Read the model definition and answer for the solid it produces. Units are mm, in the model's axes. Coordinates: 2 decimals unless noted, no trailing zeros. Loops run counter-clockwise (first coordinate to the right, second up) from the corner with the lowest first, then second, coordinate; pieces in that order, holes last. Notation, with made-up numbers: (-24.5, 24.5) -> (-17.5, 24.5) arc R37 cw to (-17.5, 61.5) -> close; hole circle Ø3 at (24, -11.75). An arc over 180 degrees is marked (long way). Answer as a JSON object with one key per item and string values. Group by question number.
1) Section D-D, the plane x = 25 is taken. Give the vertices of the cut face in (y, z).
2) Consider probe 1 along Y at (x, z) = (0, 5.75); probe 2 along Y at (x, z) = (25, 4); probe 3 along X at (y, z) = (5, 4). Determine where each line is inside the solid, lowest interval first. Write a range as [from, to].
3) Section C-C, the plane y = 2 is taken. Give the vertices of the cut face in (x, z), plus the area to 3 significant figures.
4) Section A-A, the plane z = 4.25 is taken. Give the vertices of the cut face in (x, y).
5) Flat-ended cylindrical pins translate along their axes: P1, Ø8, axis at x = 25, y = 0, coming from the -Z side; P2, Ø5.5, axis at x = -25, y = 0, coming from the +Z side. Find the tip coordinate at first contact, or state that the pin passes through.
6) Section B-B, the plane x = 0 is taken. Give the vertices of the cut face in (y, z).
7) Determine the mould class of faces 1 (the face through (22, 0, 6)), 2 (the face through (-35, 0, 6)), 3 (the face through (0, -19, 6)), 4 (the face through (0, 19, 6)) for opening direction Y: released by +Y, released by -Y, zero draft, split by the parting line, or undercut.
from build123d import *

# Parameters (mm, degrees)
CYLINDER004_R     = 7.5
CYLINDER004_DEPTH = 10
CYLINDER003_R     = 3
CYLINDER003_DEPTH = 10
ARRAY001_X_COUNT  = 2
ARRAY001_X_PITCH  = 50
RECTANGLE001_W    = 70
RECTANGLE001_H    = 38
EXTRUDE001_DEPTH  = 10


with BuildPart() as cilindro004:
    # Cylinder004 → Cylinder004 (new body)
    with BuildSketch(Plane(origin=(0, -5, 0), x_dir=(1, 0, 0), z_dir=(0, 0, 1))):
        Circle(CYLINDER004_R)
    extrude(amount=CYLINDER004_DEPTH)


with BuildPart() as fusion:
    # Cylinder003 → Cylinder003 (new body)
    with BuildSketch(Plane(origin=(25, -5, 0), x_dir=(1, 0, 0), z_dir=(0, 0, 1))):
        Circle(CYLINDER003_R)
    extrude(amount=CYLINDER003_DEPTH)

    # Array001 X: Fusion ×2


with BuildPart() as fusion_1:
    add(fusion.part)
    with Locations(*[(-i * ARRAY001_X_PITCH, 0, 0) for i in range(1, ARRAY001_X_COUNT)]):
        add(fusion.part)

    # Fusion: union Cilindro004
    add(cilindro004.part)


with BuildPart() as obj1:
    # Rectangle001 → Extrude001 (new body)
    with BuildSketch(Plane(origin=(-35, -24, 0), x_dir=(1, 0, 0), z_dir=(0, 0, 1))):
        with Locations((35, 19)):
            Rectangle(RECTANGLE001_W, RECTANGLE001_H)
    extrude(amount=EXTRUDE001_DEPTH)

    # Cut003: cut Fusion
    add(fusion_1.part, mode=Mode.SUBTRACT)


with BuildPart() as obj1_1:
    # Cut003 placement: moved
    add(obj1.part.moved(Location((0, 5, 1))))


solid = obj1_1.part
Determined:
{
 "1": {"outline": "(-19, 1) -> (-3, 1) -> (-3, 11) -> (-19, 11) -> close; (3, 1) -> (19, 1) -> (19, 11) -> (3, 11) -> close"},
 "2": {"probe 1": "[-19, -7.5], [7.5, 19]", "probe 2": "[-19, -3], [3, 19]", "probe 3": "[-35, -5.59], [5.59, 35]"},
 "3": {"outline": "(-35, 1) -> (-27.24, 1) -> (-27.24, 11) -> (-35, 11) -> close; (-22.76, 1) -> (-7.23, 1) -> (-7.23, 11) -> (-22.76, 11) -> close; (7.23, 1) -> (22.76, 1) -> (22.76, 11) -> (7.23, 11) -> close; (27.24, 1) -> (35, 1) -> (35, 11) -> (27.24, 11) -> close", "area": "466 mm²"},
 "4": {"outline": "(-35, -19) -> (35, -19) -> (35, 19) -> (-35, 19) -> close; hole circle Ø6 at (-25, 0); hole circle Ø15 at (0, 0); hole circle Ø6 at (25, 0)"},
 "5": {"P1": "z = 1", "P2": "through"},
 "6": {"outline": "(-19, 1) -> (-7.5, 1) -> (-7.5, 11) -> (-19, 11) -> close; (7.5, 1) -> (19, 1) -> (19, 11) -> (7.5, 11) -> close"},
 "7": {"face 1": "undercut", "face 2": "zero draft", "face 3": "released by -Y", "face 4": "released by +Y"}
}
